```python
from build123d import *

# Parameters (mm, degrees)
ESQUISSE1_W             = 58
ESQUISSE1_H             = 8
BOSS_EXTRU_1_DEPTH      = 50
ESQUISSE2_R             = 15
ESQUISSE2_R_2           = 13
ENL_V_MAT_EXTRU_1_DEPTH = 5
ESQUISSE3_R             = 1.5
ENL_V_MAT_EXTRU_2_DEPTH = 10
ESQUISSE4_R             = 1.5
ENL_V_MAT_EXTRU_3_DEPTH = 10
ESQUISSE5_R             = 1.5
ENL_V_MAT_EXTRU_4_DEPTH = 51


with BuildPart() as part:
    # Esquisse1 → Boss.-Extru.1 (new body)
    with BuildSketch(Plane.XY):
        with Locations((23.5, -49)):
            Rectangle(ESQUISSE1_W, ESQUISSE1_H)
    extrude(amount=BOSS_EXTRU_1_DEPTH)

    # Esquisse2 → Enlèv. mat.-Extru.1 (cut)
    with BuildSketch(Plane(origin=(0, -45, 0), x_dir=(-1, 0, 0), z_dir=(0, 1, 0))):
        with Locations((-24.5, 25)):
            Circle(ESQUISSE2_R)
        with Locations((-24.5, 25)):
            Circle(ESQUISSE2_R_2, mode=Mode.SUBTRACT)
    extrude(amount=-ENL_V_MAT_EXTRU_1_DEPTH, mode=Mode.SUBTRACT)

    # Esquisse3 → Enlèv. mat.-Extru.2 (cut)
    with BuildSketch(Plane.ZY.offset(5.5)):
        with Locations((12.5, -47.5)):
            Circle(ESQUISSE3_R)
        with Locations((37.5, -47.5)):
            Circle(ESQUISSE3_R)
    extrude(amount=-ENL_V_MAT_EXTRU_2_DEPTH, mode=Mode.SUBTRACT)

    # Esquisse4 → Enlèv. mat.-Extru.3 (cut)
    with BuildSketch(Plane(origin=(52.5, 0, 0), x_dir=(0, 0, -1), z_dir=(1, 0, 0))):
        with Locations((-37.5, -47.5)):
            Circle(ESQUISSE4_R)
        with Locations((-12.5, -47.5)):
            Circle(ESQUISSE4_R)
    extrude(amount=-ENL_V_MAT_EXTRU_3_DEPTH, mode=Mode.SUBTRACT)

    # Esquisse5 → Enlèv. mat.-Extru.4 (cut, through all)
    with BuildSketch(Plane(origin=(0, 0, 0), x_dir=(-1, 0, 0), z_dir=(0, 0, -1))):
        with Locations((-23.5, -47.5)):
            Circle(ESQUISSE5_R)
    extrude(amount=-ENL_V_MAT_EXTRU_4_DEPTH, mode=Mode.SUBTRACT)


solid = part.part
```
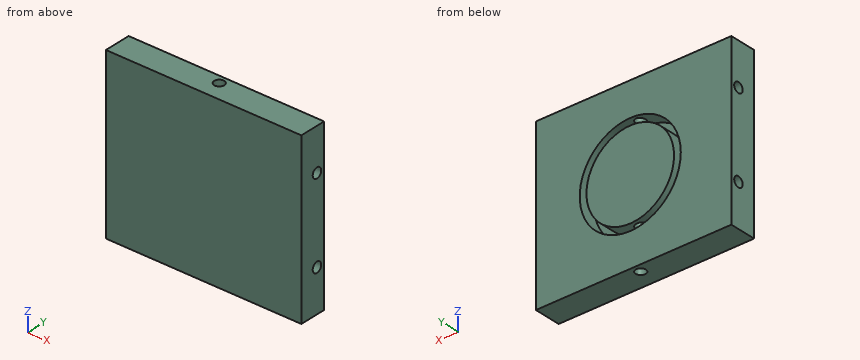
Work out the finished part from the listing and answer in its coordinate system (mm). Give positions to 0.01 mm unless a question says otherwise; leave off trailing zeros. Order: outer loops, then holes, each group sorted by start corner. A loop starts at its lowest first (then second) coordinate and runs counter-clockwise, first axis right, second up.
1. Section A-A, the plane y = -47.5 is taken. Give the number of separate pieces and of enclosed holes in the cut face, and give its area (3 significant figures).
Result sheet:
separate pieces: 4
enclosed holes: 0
area: 2,470 mm2
2. Section D-D, the plane x = 33.5 is taken. Determine the outline of the cut face in (y, z).
Result sheet:
outline: (-53, 0) - (-45, 0) - (-45, 13) - (-50, 13) - (-50, 15.62) - (-45, 15.62) - (-45, 34.38) - (-50, 34.38) - (-50, 37) - (-45, 37) - (-45, 50) - (-53, 50) - close
3. This flat-tipped pin is pushed along its axis until it touches: P1, Ø1, axis at y = -47, z = 12.5, coming from the -X side. Where does it stop, or does it pass through?
Result sheet:
P1: stops at x = 4.5
4. Section B-B, the plane z = 25 is taken. Determine the outline of the cut face in (x, y).
Result sheet:
outline: (-5.5, -53) - (52.5, -53) - (52.5, -45) - (39.5, -45) - (39.5, -50) - (37.5, -50) - (37.5, -45) - (11.5, -45) - (11.5, -50) - (9.5, -50) - (9.5, -45) - (-5.5, -45) - close; hole circle Ø3 at (23.5, -47.5)
5. Straight lines are drawn through the part: L1, parallel to X at y = -47.5, z = 46.75; L2, parallel to Y at x = 46.5, z = 37.5; L3, parallel to X at y = -45.25, z = 29. For each, find the intervals that lie inside material, in ascending order.
Result sheet:
L1: x = -5.5 to 22, 25 to 52.5
L2: y = -53 to -49, -46 to -45
L3: x = -5.5 to 10.04, 12.13 to 36.87, 38.96 to 52.5
6. Section C-C, the plane x = 1 is taken. Determine the outline of the cut face in (y, z), and give its area (3 significant figures).
Result sheet:
outline: (-53, 0) - (-45, 0) - (-45, 50) - (-53, 50) - close; hole circle Ø3 at (-47.5, 12.5); hole circle Ø3 at (-47.5, 37.5)
area: 386 mm2
